Autodesk Inventor part; units mm, degrees
ref_plane "YZ Plane" through (0, 0, 0) normal (1, 0, 0) x (0, 1, 0)
ref_plane "XZ Plane" through (0, 0, 0) normal (0, 1, 0) x (-1, 0, 0)
ref_plane "XY Plane" through (0, 0, 0) normal (0, 0, 1) x (1, 0, 0)
sketch "Sketch7" plane through (0, 0, 0) normal (0, 0, 1) x (1, 0, 0)
  line L0 (0, 0) -> (70, 0)
  line L1 (70, 0) -> (70, 30)
  line L2 (70, 30) -> (0, 30)
  line L3 (0, 30) -> (0, 0)
  dimension "d25" = 70
  dimension "d26" = 30
extrude "Extrusion5" add sketch "Sketch7" against normal blind 150
sketch "Sketch8" plane through (0, 30, 0) normal (0, 1, 0) x (1, 0, 0)
  line L0 (0, 0) -> (3, 0)
  line L1 (3, 0) -> (3, 3)
  line L2 (3, 3) -> (0, 3)
  line L3 (0, 3) -> (0, 0)
  line L4 (70, 150) -> (67, 150)
  line L5 (67, 150) -> (67, 147)
  line L6 (67, 147) -> (70, 147)
  line L7 (70, 147) -> (70, 150)
  line L8 (3, 3) -> (67, 3)
  line L9 (67, 3) -> (67, 147)
  line L10 (67, 147) -> (3, 147)
  line L11 (3, 147) -> (3, 3)
  dimension "d29" = 3
  dimension "d30" = 3
  dimension "d31" = 3
  dimension "d32" = 3
extrude "Extrusion6" cut sketch "Sketch8" against normal blind 27 contours L11 L10 L9 L8
sketch "Sketch10" plane through (0, 0, -150) normal (0, 0, -1) x (-1, 0, 0)
  line L0 (-70, 30) -> (-70, 0)
  line L1 (-70, 0) -> (-61.5, 0)
  line L2 (-70, 4) -> (-70, 0)
  line L3 (0, 0) -> (0, 30)
  line L4 (0, 0) -> (-8.5, 0)
  line L5 (0, 4) -> (0, 0)
  line L6 (-54.5, 4) -> (-41.5, 4)
  line L7 (-61.5, 0) -> (-51.709, 0)
  line L8 (-8.5, 0) -> (-41.5, 0)
  line L9 (-26.0357, 0) -> (-23.5, 0)
  line L10 (-40.5, 4) -> (-40.5, 30)
  line L11 (-40.5, 30) -> (-55.5, 30)
  line L12 (-55.5, 30) -> (-55.5, 4)
  line L13 (-70, 0) -> (0, 0)
  line L14 (-55.5, 0) -> (-40.5, 0)
  line L15 (-55.5, 4) -> (-40.5, 4)
  line L16 (-11.5, 4) -> (-11.5, 30)
  line L17 (-11.5, 30) -> (-26.5, 30)
  line L18 (-26.5, 30) -> (-26.5, 4)
  line L19 (-26.5, 4) -> (-11.5, 4)
  point P0 (-48, 10)
  dimension "d188" = 15
  dimension "d189" = 15
sketch "Sketch15" plane through (0, 0, -150) normal (0, 0, -1) x (-1, 0, 0)
  line L0 (-70, 30) -> (-70, 0)
  line L1 (0, 30) -> (0, 0)
  line L2 (-70, 30) -> (0, 30)
  line L3 (0, 30) -> (0, 18)
  line L4 (0, 18) -> (-70, 18)
  line L5 (-70, 18) -> (-70, 30)
  dimension "d100" = 12
extrude "Extrusion10" cut sketch "Sketch15" against normal blind 10000
sketch "Sketch20" plane through (67, 3, -147) normal (-1, 0, 0) x (0, 0, 1)
  line L0 (0, 15) -> (144, 15)
  line L1 (144, 15) -> (144, 12)
  line L2 (144, 12) -> (0, 12)
  line L3 (0, 12) -> (0, 15)
  line L4 (0, 12) -> (2, 12)
  line L5 (2, 12) -> (2, 11)
  line L6 (2, 11) -> (0, 11)
  line L7 (0, 11) -> (0, 12)
  line L8 (144, 12) -> (142, 12)
  line L9 (142, 12) -> (142, 11)
  line L10 (142, 11) -> (144, 11)
  line L11 (144, 11) -> (144, 12)
  point P0 (147, -3)
  point P1 (2, 12)
  dimension "d132" = 144
  dimension "d133" = 3
  dimension "d134" = 2
  dimension "d135" = 1
  dimension "d136" = 2
  dimension "d137" = 1
extrude "Extrusion17" cut sketch "Sketch20" against normal blind 1 contours L2 L5 L6 L7 | L11 L10 L9 L2
sketch "Sketch21" plane through (70, 0, 0) normal (1, 0, 0) x (0, 0, -1)
  line L0 (0, 0) -> (0, 18)
  line L1 (0, 18) -> (10, 18)
  line L2 (10, 18) -> (10, 15)
  line L3 (10, 15) -> (0, 15)
  line L4 (0, 15) -> (0, 18)
  line L5 (139.9948, 18) -> (149.9948, 18)
  line L6 (149.9948, 18) -> (149.9948, 15)
  line L7 (149.9948, 15) -> (139.9948, 15)
  line L8 (139.9948, 15) -> (139.9948, 18)
  dimension "d144" = 10
  dimension "d145" = 3
  dimension "d146" = 10
  dimension "d147" = 3
extrude "Extrusion18" add sketch "Sketch21" along normal blind 5
sketch "Sketch23" plane through (0, 0, -150) normal (-1, 0, 0) x (0, 0, 1)
  line L0 (150, 18) -> (147, 18)
  line L1 (150, 18) -> (140, 18)
  line L2 (140, 18) -> (140, 15)
  line L3 (140, 15) -> (150, 15)
  line L4 (150, 15) -> (150, 18)
  line L5 (9.9944, 18) -> (-0.0056, 18)
  line L6 (-0.0056, 18) -> (-0.0056, 15)
  line L7 (-0.0056, 15) -> (9.9944, 15)
  line L8 (9.9944, 15) -> (9.9944, 18)
  point P0 (150, 0)
  point P1 (149.4, 18)
  point P2 (149.4, 18)
  dimension "d158" = 10
  dimension "d159" = 3
  dimension "d160" = 10
  dimension "d161" = 3
extrude "Extrusion20" add sketch "Sketch23" along normal blind 5
sketch "Sketch25" plane through (3, 18, -147) normal (0, 1, 0) x (1, 0, 0)
  line L0 (72, -147) -> (-8, -147)
  line L1 (-8, -147) -> (-5.5, -147)
  line L2 (-8, -142) -> (-8, -147)
  line L3 (53.15, -147) -> (72, -147)
  line L4 (72, -147) -> (69.5, -147)
  line L5 (72, -142) -> (72, -147)
  line L6 (72, 2.9948) -> (69.5, 2.9948)
  line L7 (72, -2.0052) -> (72, 2.9948)
  line L8 (-8, 3.0056) -> (-8, -6.9944)
  line L9 (-8, 3.0056) -> (-5.5, 3.0056)
  line L10 (-8, -1.9944) -> (-8, 3.0056)
  circle A0 centre (-5.5, -1.9944) radius 1.5
  circle A1 centre (69.5, -2.0052) radius 1.5
  circle A2 centre (69.5, -142) radius 1.5
  circle A3 centre (-5.5, -142) radius 1.5
  point P0 (-3, -147)
  point P1 (10.85, -147)
  dimension "d180" = 3
  dimension "d181" = 3
  dimension "d182" = 3
  dimension "d183" = 3
extrude "Extrusion22" cut sketch "Sketch25" against normal blind 10
extrude "Extrusion23" cut sketch "Sketch10" against normal blind 10
sketch "Sketch26" plane through (0, 3, 0) normal (0, 1, 0) x (1, 0, 0)
  line L0 (3, 147) -> (67, 147)
  line L1 (3, 147) -> (13, 147)
  line L2 (3, 132.7) -> (3, 147)
  line L3 (61.5, 121.8573) -> (13, 121.8573)
  line L4 (16.5, 91.8787) -> (44.5, 91.8787)
  circle A0 centre (16.5, 81.9) radius 2.25
  circle A1 centre (44.5, 81.9) radius 2.25
  circle A2 centre (61.5, 132.7) radius 2.25
  circle A3 centre (13, 132.7) radius 2.25
  point P0 (0, 0)
  dimension "d195" = 48.5
  dimension "d200" = 28
  dimension "d233" = 4.5
  dimension "d234" = 4.5
  dimension "d235" = 4.5
  dimension "d236" = 4.5
fillet "Face Fillet3" radius 5.5 1 edges at (70, 0, -75)
fillet "Face Fillet4" radius 5.5 1 edges at (0, 0, -75)
sketch "Sketch27" plane through (0, 0, 0) normal (0, 0, 1) x (1, 0, 0)
  line L0 (12.25, 28.2) -> (57.75, 28.2)
  line L1 (57.75, 28.2) -> (57.75, 7.8)
  line L2 (57.75, 7.8) -> (12.25, 7.8)
  line L3 (12.25, 7.8) -> (12.25, 28.2)
  line L4 (75, 18) -> (-5, 18)
  line L5 (57.75, 28.2) -> (12.25, 7.8) construction
  line L6 (12.25, 7.8) -> (12.75, 7.8)
  line L7 (12.25, 8.3) -> (12.25, 7.8)
  line L8 (57.75, 7.8) -> (57.25, 7.8)
  line L9 (57.75, 8.3) -> (57.75, 7.8)
  circle A0 centre (14.1, 9.65) radius 1.35
  line L10 (15.95, 7.8) -> (15.45, 7.8)
  circle A1 centre (55.9, 9.65) radius 1.35
  line L11 (57.75, 8.3) -> (57.75, 7.8)
  point P0 (0, 0)
  point P1 (35, 18)
  dimension "d210" = 45.5
  dimension "d211" = 20.4
  dimension "d218" = 2.7
  dimension "d219" = 0.5
  dimension "d221" = 2.7
  dimension "d223" = 0.5
extrude "Extrusion27" cut sketch "Sketch27" against normal blind 10 contours A0 | A1
sketch "Sketch28" plane through (0, 3, 0) normal (0, 1, 0) x (1, 0, 0)
  line L0 (51.8999, 76.8126) -> (11.6522, 76.8126)
  line L1 (11.6522, 76.8126) -> (11.6522, 60.3126)
  line L2 (51.8999, 60.3126) -> (51.8999, 76.8126)
  line L3 (51.8999, 58.2305) -> (51.8999, 60.3126)
  circle A0 centre (47.6999, 60.3126) radius 2.25
  line L4 (11.6522, 57.5365) -> (11.6522, 60.3126)
  circle A1 centre (15.8522, 60.3126) radius 2.25
  point P0 (0, 0)
  dimension "d226" = 16.5
  dimension "d228" = 4.5
  dimension "d230" = 4.5
extrude "Extrusion28" cut sketch "Sketch28" against normal blind 10
extrude "Extrusion29" cut sketch "Sketch26" against normal blind 10
properties part number "BOT_HOLDER_ENGR-2200_3DPrint"
Verification items for the finished model (mm, model axes). A direction names the side the tool comes from. Coordinates: 2 decimals unless noted, no trailing zeros. Order: outer loops, then holes, each group sorted by start corner. A loop starts at its lowest first (then second) coordinate and runs counter-clockwise, first axis right, second up. Notation, with made-up numbers: (51, 48.25) -> (84, 48.25) arc R12 cw to (84, 62.25) -> close; hole circle Ø1 at (64, 66). An arc over 180 degrees is marked (long way). Put each result on its own line as item: value. Start each with the question number.
1. Cross-section at B-B, the plane x = 72.5. Record the boundary of the cut face in (y, z), then the cut area to 3 significant figures.
2. Cross-section at A-A, the plane z = -132.7. Record the boundary of the cut face in (x, y), then the cut area to 3 significant figures.
3. Access from +Z, -Z, +X, -X, +Y, -Y to the whole of each face (thin tool, end or side, straight path). Record for faces 1 (the flat face through (72, 17, -10)), 2 (the flat face through (11.5, 11, -149)), 3 (the flat face through (-1, 15, -146)).
4. Go/stop test with flat-tipped pins: pin 1 Ø2.5 at (y, z) = (8.5, -148.5) entering from +X; pin 2 Ø10 at (x, y) = (19, 12) entering from -Z; pin 3 Ø0.8 at (y, z) = (14.5, -3.5) entering from -X. Record where each tip stops, or that it passes through.
5. Cross-section at D-D, the plane z = -72. Record the boundary of the cut face in (x, y).
6. Cross-section at C-C, the plane x = 61. Record the boundary of the cut face in (y, z), then the cut area to 3 significant figures.
7. Material ranges on L1, parallel to Z at x = -2.5, y = 16.1; L2, parallel to Y at x = 14, z = -1; L3, parallel to Z at x = 7.5, y = 15, recorded low to high. Write a range as [from, to].
8. Mould release check, pull along Z, two halves, no side actions. Record for faces 4 (the flat face through (-2, 17, -10)), 5 (the flat face through (-2, 17, -150.006)), 6 (the flat face through (-1, 15, -6)): released by +Z, released by -Z, zero draft, split by the parting line, or undercut.
Computed:
1. outline: (15, -149.99) -> (18, -149.99) -> (18, -146.49) -> (15, -146.49) -> close; (15, -143.49) -> (18, -143.49) -> (18, -139.99) -> (15, -139.99) -> close; (15, -10) -> (18, -10) -> (18, -6.5) -> (15, -6.5) -> close; (15, -3.5) -> (18, -3.5) -> (18, 0) -> (15, 0) -> close
1. area: 42.0 mm2
2. outline: (0, 5.5) arc R5.5 ccw to (5.5, 0) -> (10.75, 0) -> (10.75, 3) -> (3, 3) -> (3, 18) -> (0, 18) -> close; (15.25, 0) -> (59.25, 0) -> (59.25, 3) -> (15.25, 3) -> close; (63.75, 0) -> (64.5, 0) arc R5.5 ccw to (70, 5.5) -> (70, 18) -> (67, 18) -> (67, 3) -> (63.75, 3) -> close
2. area: 260 mm2
3. face 1: +X, +Y, -Y
3. face 2: -Z, +Y
3. face 3: +Z, -Z, -X, -Y
4. pin 1: x = 70
4. pin 2: z = -3
4. pin 3: x = 0
5. outline: (0, 5.5) arc R5.5 ccw to (5.5, 0) -> (64.5, 0) arc R5.5 ccw to (70, 5.5) -> (70, 18) -> (67, 18) -> (67, 3) -> (3, 3) -> (3, 18) -> (0, 18) -> close
6. outline: (0, -150) -> (18, -150) -> (18, -147) -> (3, -147) -> (3, -134.89) -> (0, -134.89) -> close; (0, -130.51) -> (3, -130.51) -> (3, -3) -> (18, -3) -> (18, 0) -> (0, 0) -> close
6. area: 527 mm2
7. L1: [-150.01, -146.51], [-143.51, -140.01], [-10, -6.5], [-3.5, 0]
7. L2: [0, 8.3], [11, 18]
7. L3: [-150, -147], [-3, 0]
8. face 4: undercut
8. face 5: released by -Z
8. face 6: zero draft
